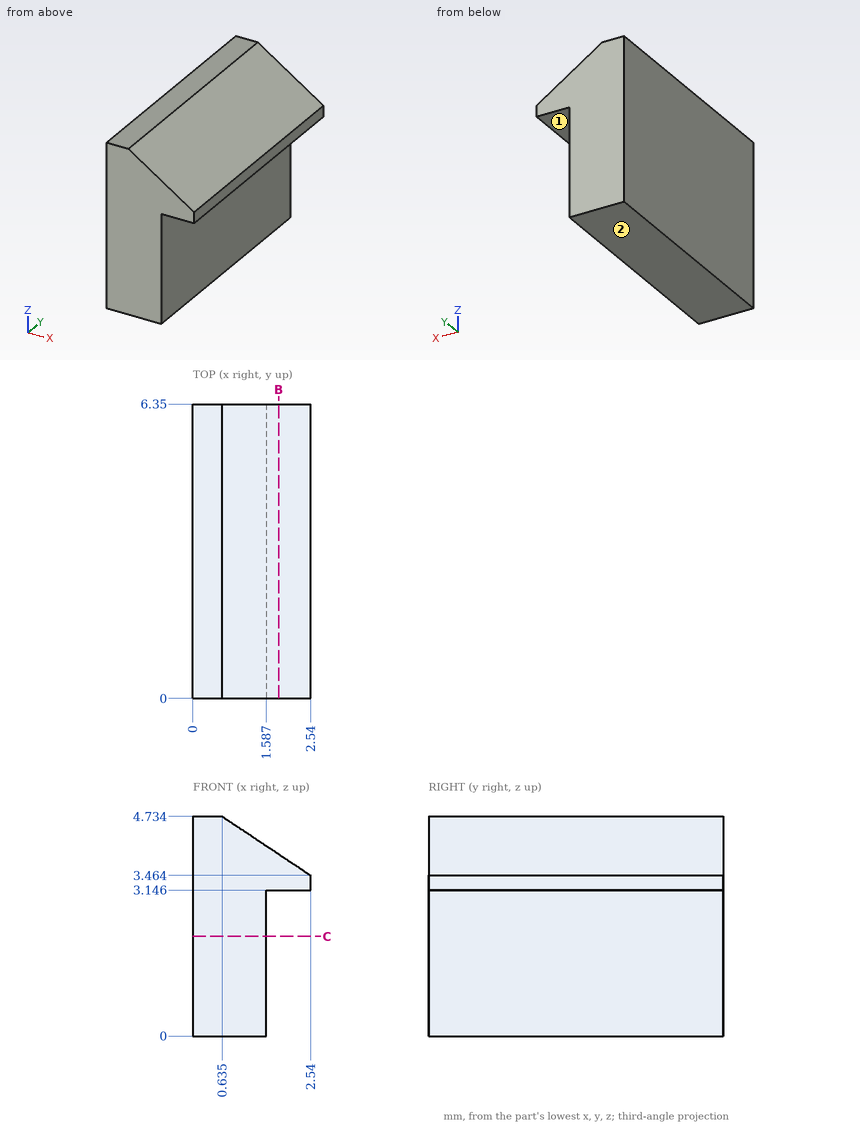
Geometry: see drawing. Coordinates: mm, zero at the bounding-box minimum. A direction names the side the tool comes from. Give positions to 0.01 mm unless a question says otherwise; leave off trailing zeros. Order: outer loops, then holes, each group sorted by start corner. A loop starts at its lowest first (then second) coordinate and runs counter-clockwise, first axis right, second up. Notation, with made-up numbers: M -28.75,-3.75 L 12.25,-3.75 A15 ccw 12.25,0.25 Z; hole C -18,59 d4. An arc over 180 degrees is marked long. Answer as CSV lines item,"result". Start each with the question number.
1) Cut plane C-C (z = 2.15). Output: boundary loops of the cut face in (x, y), then the cut area to 3 significant figures.
2) Cut plane B-B (x = 1.85). Output: boundary loops of the cut face in (y, z).
3) First-contact query: P1, Ø2, axis at y = 4.5, z = 1.5, coming from the -X side. Flat tip, straight axial feed; report the tip coordinate or a pass-through.
4) Set-up query: the marked faces 1 and 2. Return all of +Z, -Z, +X, -X, +Y, -Y with unobstructed straight access to the full face (end or side cutting, diameter ignored); none if empty.
5) Line query: line 1 (X direction, y = 3.5, z = 1.65); line 2 (X direction, y = 4.5, z = 3.6) (1 decimal); line 3 (Z direction, x = 1.1, y = 3.25) (1 decimal). Output: solid intervals per line, ascending. Write a range as from..to.
Findings below:
1,outline,"M 0,0 L 1.59,0 L 1.59,6.35 L 0,6.35 Z"
1,area,"10.1 mm²"
2,outline,"M 0,3.15 L 6.35,3.15 L 6.35,3.92 L 0,3.92 Z"
3,P1,"stops at x = 0"
4,face 1,"-Z, +X, +Y, -Y"
4,face 2,"-Z, +X, -X, +Y, -Y"
5,line 1,"x = 0..1.59"
5,line 2,"x = 0..2.3"
5,line 3,"z = 0..4.4"
